```python
from build123d import *

# Parameters (mm, degrees)
SKETCH_1_W          = 136
SKETCH_1_H          = 104
EXTRUDE_1_DEPTH     = 42
SKETCH_2_W          = 116
SKETCH_2_H          = 84
CUT_EXTRUDE_1_DEPTH = 36
SKETCH_6_R          = 2.2
CUT_EXTRUDE_5_DEPTH = 136


with BuildPart() as part:
    # 草图1 → 凸台-拉伸1 (new body)
    with BuildSketch(Plane(origin=(0, 0, 0), x_dir=(1, 0, 0), z_dir=(0, 1, 0))):
        Rectangle(SKETCH_1_W, SKETCH_1_H)
    extrude(amount=EXTRUDE_1_DEPTH)

    # 草图2 → 切除-拉伸1 (cut)
    with BuildSketch(Plane(origin=(0, 42, 0), x_dir=(1, 0, 0), z_dir=(0, 1, 0))):
        Rectangle(SKETCH_2_W, SKETCH_2_H)
    extrude(amount=-CUT_EXTRUDE_1_DEPTH, mode=Mode.SUBTRACT)

    # 草图6 → 切除-拉伸5 (cut)
    with BuildSketch(Plane.ZY.offset(68)):
        with Locations((-26, 21)):
            Circle(SKETCH_6_R)
        with Locations((26, 21)):
            Circle(SKETCH_6_R)
        with Locations((0, 21)):
            Circle(SKETCH_6_R)
    extrude(amount=-CUT_EXTRUDE_5_DEPTH, mode=Mode.SUBTRACT)


solid = part.part
```
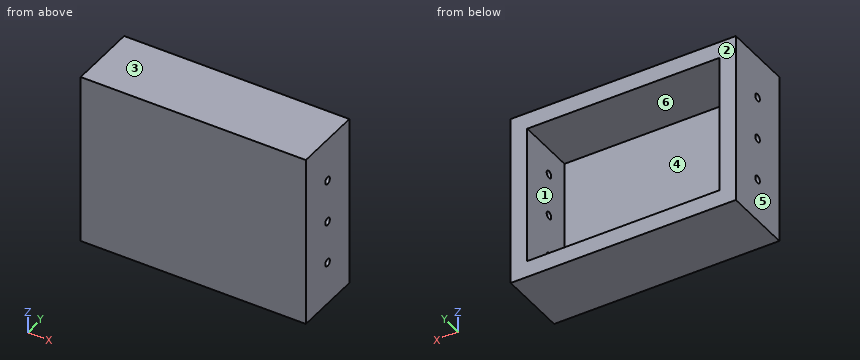
Source: CAD feature listing. Evaluate the final solid. Frame: model axes, mm. Face numbers are marked on the shaded views. A direction names the side the tool comes from. Round coordinates to 2 decimals unless told otherwise and drop trailing zeros. Loops run counter-clockwise (first coordinate to the right, second up) from the corner with the lowest first, then second, coordinate; pieces in that order, holes last.
(1) Section query A-A (y = 21). Give the number of separate pieces and of enclosed holes in the cut face, and give its area (3 significant figures).
From the geometry:
separate pieces: 6
enclosed holes: 0
area: 4,140 mm2
(2) Contact query for flat-ended pins moving along their axis: pin 1 Ø3 at (x, z) = (-12.5, -29) entering from +Y; pin 2 Ø5 at (y, z) = (21, -26) entering from -X. Output: stop coordinate, or through.
From the geometry:
pin 1: stops at y = 6
pin 2: stops at x = -68
(3) Pull-direction query (Z, two-part tool) for the marked faces 1, 2, 3 and 4; classes: +Z half, -Z half, draft (parallel to the pull), parting line (faces both ways), or undercut.
From the geometry:
face 1: undercut
face 2: draft
face 3: +Z half
face 4: undercut
(4) Section query D-D (x = -51.5). Output: boundary loops of the cut face in (y, z).
From the geometry:
outline: (0, -52) - (42, -52) - (42, -42) - (6, -42) - (6, 42) - (42, 42) - (42, 52) - (0, 52) - close
(5) Section query C-C (y = 37). Output: boundary loops of the cut face in (x, z).
From the geometry:
outline: (-68, -52) - (68, -52) - (68, 52) - (-68, 52) - close; hole (-58, -42) - (58, -42) - (58, 42) - (-58, 42) - close
(6) Material intervals for probe 1 along X at (y, z) = (35, 30); probe 2 along Z at (x, y) = (39, 14.5); probe 3 along Y at (x, z) = (-64, 0), sorted ascending.
From the geometry:
probe 1: x = -68 to -58, 58 to 68
probe 2: z = -52 to -42, 42 to 52
probe 3: y = 0 to 18.8, 23.2 to 42
(7) Section query B-B (z = 0). Output: boundary loops of the cut face in (x, y), and give its area (3 significant figures).
From the geometry:
outline: (-68, 0) - (68, 0) - (68, 18.8) - (58, 18.8) - (58, 6) - (-58, 6) - (-58, 18.8) - (-68, 18.8) - close; (-68, 23.2) - (-58, 23.2) - (-58, 42) - (-68, 42) - close; (58, 23.2) - (68, 23.2) - (68, 42) - (58, 42) - close
area: 1,450 mm2
(8) Access query for the marked faces 5 and 6. Directions: +Z, -Z, +X, -X, +Y, -Y. A direction counts if a zero-diameter tool reaches every point of the face in a straight line with its end or side. Return the directions, or none.
From the geometry:
face 5: +Z, -Z, -X, +Y, -Y
face 6: +Y
